Autodesk Inventor part; units mm, degrees
ref_plane "YZ Plane" through (0, 0, 0) normal (1, 0, 0) x (0, 1, 0)
ref_plane "XZ Plane" through (0, 0, 0) normal (0, 1, 0) x (-1, 0, 0)
ref_plane "XY Plane" through (0, 0, 0) normal (0, 0, 1) x (1, 0, 0)
sketch "Sketch51" plane through (0, 0, 0) normal (0, 1, 0) x (-1, 0, 0)
  line L0 (1.3484, 37.0338) -> (-3.7316, 37.0338)
  line L1 (-3.7316, 37.0338) -> (-3.7316, -191.5662)
  line L2 (-3.7316, -191.5662) -> (1.3484, -191.5662)
  line L3 (1.3484, -191.5662) -> (1.3484, 37.0338)
  point P0 (0, 0)
  dimension "d172" = 5.08
  dimension "d173" = 228.6
extrude "Extrusion37" add sketch "Sketch51" along normal blind 71.12
sketch "Sketch52" plane through (-1.3484, 0, 37.0338) normal (0, 0, 1) x (1, 0, 0)
  line L0 (5.08, 0) -> (5.08, 71.12)
  line L1 (5.08, 71.12) -> (-24.13, 71.12)
  line L2 (-24.13, 71.12) -> (-24.13, 66.04)
  line L3 (-24.13, 66.04) -> (5.08, 66.04)
  line L4 (5.08, 66.04) -> (5.08, 71.12)
  point P0 (1.3484, 0)
  dimension "d176" = 5.08
  dimension "d177" = 29.21
extrude "Extrusion38" add sketch "Sketch52" against normal blind 228.6
sketch "Sketch54" plane through (0, 0, 0) normal (0, -1, 0) x (1, 0, 0)
  line L0 (-20.3984, 37.0338) -> (-141.0484, 37.0338)
  line L1 (-141.0484, 37.0338) -> (-141.0484, -191.5662)
  line L2 (-141.0484, -191.5662) -> (-20.3984, -191.5662)
  line L3 (-20.3984, -191.5662) -> (-20.3984, 37.0338)
  line L4 (-25.4784, 37.0338) -> (-1.3484, 37.0338)
  line L5 (-1.3484, -191.5662) -> (-25.4784, -191.5662)
  line L6 (-1.3484, -191.5662) -> (-1.3484, 37.0338)
  point P0 (0, 0)
  dimension "d180" = 0
  dimension "d181" = 0
  dimension "d182" = 19.05
  dimension "d183" = 120.65
extrude "Extrusion39" add sketch "Sketch54" against normal blind 5.08 contours L3 L2 L1 L0
sketch "Sketch55" plane through (-1.3484, 0, 37.0338) normal (0, 0, 1) x (1, 0, 0)
  line L0 (-139.7, 5.08) -> (-19.05, 5.08)
  line L1 (-24.13, 66.04) -> (-24.13, 71.12)
  line L2 (-19.05, 5.08) -> (-24.13, 5.08)
  line L3 (-24.13, 5.08) -> (-24.13, 71.12)
  line L4 (-24.13, 71.12) -> (-19.05, 71.12)
  line L5 (-19.05, 71.12) -> (-19.05, 5.08)
  point P0 (1.3484, 0)
extrude "Extrusion40" add sketch "Sketch55" against normal blind 228.6
sketch "Sketch56" plane through (3.7316, 0, 37.0338) normal (0, 0, 1) x (1, 0, 0)
  line L0 (-29.4089, 71.12) -> (0, 71.12)
  line L1 (0, 71.12) -> (0, 0)
  line L2 (0, 0) -> (-29.4089, 0)
  line L3 (-29.4089, 0) -> (-29.4089, 71.12)
  line L4 (0, 71.12) -> (-29.21, 71.12)
  point P0 (-3.7316, 0)
  dimension "d275" = 0
extrude "Extrusion41" add sketch "Sketch56" against normal blind 5.08
sketch "Sketch57" plane through (3.7316, 0, -191.5662) normal (0, 0, -1) x (-1, 0, 0)
  line L0 (29.4089, 5.08) -> (29.4089, 71.12)
  line L1 (29.4089, 71.12) -> (0, 71.12)
  line L2 (0, 71.12) -> (0, -0.0331)
  line L3 (0, -0.0331) -> (29.4089, -0.0331)
  line L4 (29.4089, -0.0331) -> (29.4089, 71.12)
  point P0 (3.7316, 0)
extrude "Extrusion42" add sketch "Sketch57" against normal blind 5.08
sketch "Sketch58" plane through (0, 71.12, 0) normal (0, 1, 0) x (1, 0, 0)
  line L0 (-25.4784, -31.9538) -> (-25.4784, 186.4862)
  line L1 (-141.0484, 191.5662) -> (-141.0484, -37.0338)
  line L2 (-25.4784, 109.0162) -> (-141.0484, 109.0162)
  line L3 (-141.0484, 109.0162) -> (-141.0484, 147.1162)
  line L4 (-141.0484, 147.1162) -> (-25.4784, 147.1162)
  line L5 (-25.4784, 147.1162) -> (-25.4784, 109.0162)
  line L6 (-25.6773, 191.5662) -> (-141.0484, 191.5662)
  point P0 (0, 0)
  dimension "d192" = 38.1
  dimension "d193" = 44.45
extrude "Extrusion43" add sketch "Sketch58" against normal blind 5.08
sketch "Sketch59" plane through (-141.0484, 71.12, -147.1162) normal (-1, 0, 0) x (0, 0, 1)
  line L0 (0, 0) -> (0, -5.08)
  line L1 (184.15, -71.12) -> (-44.45, -71.12)
  line L2 (0, 0) -> (5.08, 0)
  line L3 (5.08, 0) -> (5.08, -71.12)
  line L4 (5.08, -71.12) -> (0, -71.12)
  line L5 (0, -71.12) -> (0, 0)
  line L6 (38.1, 0) -> (38.1, -5.08)
  line L7 (38.1, 0) -> (33.02, 0)
  line L8 (33.02, 0) -> (33.02, -71.12)
  line L9 (33.02, -71.12) -> (38.1, -71.12)
  line L10 (38.1, -71.12) -> (38.1, 0)
  point P0 (147.1162, -71.12)
  dimension "d196" = 5.08
  dimension "d197" = 5.08
extrude "Extrusion44" add sketch "Sketch59" against normal blind 120.65
sketch "Sketch60" plane through (-141.0484, 0, -191.5662) normal (-1, 0, 0) x (0, 0, 1)
  line L0 (49.53, 5.08) -> (77.47, 5.08)
  line L1 (5.08, 0) -> (223.52, 0)
  line L2 (49.53, 5.08) -> (77.4104, 5.08)
  line L3 (77.4104, 5.08) -> (77.4104, 0)
  line L4 (77.4104, 0) -> (49.53, 0)
  line L5 (49.53, 0) -> (49.53, 5.08)
  point P0 (191.5662, 0)
extrude "Extrusion45" cut sketch "Sketch60" against normal blind 120.65
sketch "Sketch61" plane through (-25.4784, 66.04, -142.0362) normal (-1, 0, 0) x (0, 0, 1)
  line L0 (0, -66.04) -> (0, 0)
  line L1 (27.94, 0) -> (27.94, -60.96)
  line L2 (27.94, 0) -> (0, 0)
  line L3 (-44.45, -66.04) -> (173.99, -66.04)
  line L4 (0, 0) -> (27.6512, 0)
  line L5 (27.6512, 0) -> (27.6512, -66.04)
  line L6 (27.6512, -66.04) -> (0, -66.04)
  line L7 (0, -66.04) -> (0, 0)
  point P0 (142.0362, -66.04)
extrude "Extrusion46" cut sketch "Sketch61" against normal blind 5.08
sketch "Sketch62" plane through (-141.0484, 5.08, -109.0162) normal (-1, 0, 0) x (0, 0, 1)
  line L0 (-33.02, -5.08) -> (-82.55, -5.08)
  line L1 (-38.1, 66.04) -> (-38.1, 0)
  line L2 (0, 66.04) -> (0, 0)
  line L3 (-5.1396, 0) -> (-5.1396, -5.08)
  line L4 (146.05, -5.08) -> (-5.1396, -5.08)
  line L5 (146.05, -5.08) -> (146.05, 0)
  line L6 (0, 0) -> (146.05, 0)
  line L7 (0, 66.04) -> (0, 0)
  line L8 (0, 66.04) -> (-38.1, 66.04)
  line L9 (-38.1, 66.04) -> (-38.1, 0)
  line L10 (-82.55, 0) -> (-38.1, 0)
  line L11 (-82.55, -5.08) -> (-82.55, 0)
  line L12 (-33.02, -5.08) -> (-82.55, -5.08)
  line L13 (-33.02, -5.08) -> (-33.02, 60.96)
  line L14 (-5.08, 60.96) -> (-33.02, 60.96)
  line L15 (-5.08, 60.96) -> (-5.08, 0)
  line L16 (0, 66.04) -> (-34.1859, 66.04)
  line L17 (-34.1859, 66.04) -> (-34.1859, -5.08)
  line L18 (-34.1859, -5.08) -> (0, -5.08)
  line L19 (0, -5.08) -> (0, 66.04)
  line L20 (-5.1396, 0) -> (-5.08, 0)
  point P0 (109.0162, -5.08)
extrude "Extrusion47" add sketch "Sketch62" against normal blind 5.08 contours L0 L17 L8 L2 L19 L4 L3 L20 L15 L14 L13 | L13 L14 L15 L20 L3 L18
sketch "Sketch63" plane through (3.7316, 0, -191.5662) normal (0, 0, -1) x (-1, 0, 0)
  line L0 (144.78, 0) -> (29.4089, 0)
  line L1 (29.4089, 5.08) -> (29.4089, 71.12)
  point P0 (3.7316, 0)
  point P1 (14.1689, 25.4)
  point P2 (0, 0)
  dimension "d206" = 25.4
  dimension "d207" = 15.24
hole "Hole8" at (-10.4373, 25.4, -191.5662) direction (0, 0, 1) diameter 3.302 end through all
sketch "Sketch64" plane through (-141.0484, 0, -191.5662) normal (-1, 0, 0) x (0, 0, 1)
  line L0 (228.6, 0) -> (0, 0)
  line L1 (44.45, 71.12) -> (44.45, 5.08)
  point P0 (191.5662, 0)
  point P1 (63.5, 25.4)
  dimension "d215" = 25.4
  dimension "d216" = 19.05
hole "Hole9" at (-141.0484, 25.4, -128.0662) direction (1, 0, 0) diameter 3.302 depth 25.4 tip angle 118.188
sketch "Sketch66" plane through (0, 71.12, 0) normal (0, 1, 0) x (1, 0, 0)
  line L0 (-141.0484, 109.0162) -> (-141.0484, 147.1162)
  line L1 (-25.4784, 109.0162) -> (-141.0484, 109.0162)
  line L2 (-141.0484, 147.1162) -> (-25.4784, 147.1162)
  point P0 (0, 0)
  point P1 (-77.5484, 137.5912)
  dimension "d227" = 9.525
hole "Hole10" at (-77.5484, 71.12, -137.5912) direction (0, -1, 0) diameter 3.81 depth 25.4 tip angle 118.188
sketch "Sketch69" plane through (-141.0484, 71.12, -109.0162) normal (0, 0, 1) x (1, 0, 0)
  line L0 (31.75, -38.1) -> (83.6211, -38.1) construction
  line L1 (31.75, -19.05) -> (83.6211, -19.05)
  line L2 (83.6211, -57.15) -> (31.75, -57.15)
  arc A0 (31.75, -19.05) -> (31.75, -57.15) centre (31.75, -38.1) ccw
  arc A1 (83.6211, -57.15) -> (83.6211, -19.05) centre (83.6211, -38.1) ccw
  line L3 (0, 0) -> (0, -66.04)
  line L4 (115.3711, -66.04) -> (115.3711, 0)
  line L5 (115.57, 0) -> (0, 0)
  point P0 (141.0484, -71.12)
  point P1 (57.6856, -38.1)
  dimension "d252" = 31.75
  dimension "d253" = 31.75
  dimension "d254" = 38.1
  dimension "d255" = 19.05
extrude "Extrusion49" cut sketch "Sketch69" against normal blind 230.1875
sketch "Sketch70" plane through (0, 71.12, 0) normal (0, 1, 0) x (1, 0, 0)
  line L0 (-20.3984, -31.9538) -> (-20.3984, 114.385)
  line L1 (-25.4784, -31.9538) -> (-25.4784, 109.0162)
  line L2 (-25.4784, 109.0162) -> (-141.0484, 109.0162)
  line L3 (-141.0484, 191.5662) -> (-141.0484, -37.0338)
  line L4 (-141.0484, -37.0338) -> (-25.6773, -37.0338)
  line L5 (-141.0484, 109.0162) -> (-141.0484, 147.1162)
  line L6 (-141.0484, 109.0162) -> (-25.6773, 109.0162)
  line L7 (-25.6773, 109.0162) -> (-25.6773, -37.0338)
  line L8 (-25.6773, -37.0338) -> (-141.0484, -37.0338)
  line L9 (-141.0484, -37.0338) -> (-141.0484, 109.0162)
  point P0 (0, 0)
extrude "Extrusion50" add sketch "Sketch70" against normal blind 15.24
sketch "Sketch71" plane through (0, 71.12, 0) normal (0, 1, 0) x (1, 0, 0)
  line L0 (-25.6773, -37.0338) -> (3.7316, -37.0338)
  line L1 (3.7316, -37.0338) -> (-155.1721, -37.0338)
  line L2 (-155.1721, -37.0338) -> (-155.1721, 120.4462)
  line L3 (-155.1721, 120.4462) -> (3.7316, 120.4462)
  line L4 (3.7316, 120.4462) -> (3.7316, -37.0338)
  point P0 (0, 0)
  dimension "d260" = 157.48
extrude "Extrusion51" cut sketch "Sketch71" against normal blind 5.08
sketch "Sketch72" plane through (0, 66.04, 0) normal (0, 1, 0) x (1, 0, 0)
  line L0 (3.7316, -37.0338) -> (3.7316, -31.9538)
  line L1 (3.7316, -37.0338) -> (-25.8998, -37.0338)
  line L2 (-25.8998, -37.0338) -> (-25.8998, 126.8083)
  line L3 (-25.8998, 126.8083) -> (3.7316, 126.8083)
  line L4 (3.7316, 126.8083) -> (3.7316, -37.0338)
  point P0 (0, 0)
extrude "Extrusion52" add sketch "Sketch72" against normal blind 5.08
sketch "Sketch73" plane through (0, 66.04, 0) normal (0, 1, 0) x (1, 0, 0)
  line L0 (-137.7579, 102.3229) -> (-23.4148, 102.3229)
  line L1 (-23.4148, 102.3229) -> (-23.4148, 125.8312)
  line L2 (-23.4148, 125.8312) -> (-137.7579, 125.8312)
  line L3 (-137.7579, 125.8312) -> (-137.7579, 102.3229)
  point P0 (0, 0)
extrude "Extrusion53" add sketch "Sketch73" against normal blind 5.08
sketch "Sketch74" plane through (0, 66.04, 0) normal (0, 1, 0) x (1, 0, 0)
  line L0 (-141.0484, -37.0338) -> (-141.0484, 120.4462)
  line L1 (-141.0484, -37.0338) -> (-52.1484, -37.0338)
  line L2 (-52.1484, -37.0338) -> (-52.1484, 64.5662)
  line L3 (-52.1484, 64.5662) -> (-141.0484, 64.5662)
  line L4 (-141.0484, 64.5662) -> (-141.0484, -37.0338)
  point P0 (0, 0)
  dimension "d267" = 88.9
  dimension "d268" = 101.6
extrude "Extrusion54" cut sketch "Sketch74" against normal blind 37.7825
sketch "Sketch76" plane through (-141.0484, 0, -191.5662) normal (-1, 0, 0) x (0, 0, 1)
  line L0 (82.55, 55.88) -> (82.55, 5.08)
  line L1 (127, 55.88) -> (82.55, 55.88)
  line L2 (82.55, 55.88) -> (127, 55.88)
  line L3 (127, 55.88) -> (82.55, 51.6083)
  line L4 (82.55, 51.6083) -> (82.55, 55.88)
  point P0 (191.5662, 0)
extrude "Extrusion55" add sketch "Sketch76" against normal blind 116.205
sketch "Sketch77" plane through (-141.0484, 0, 37.0338) normal (0, 0, 1) x (1, 0, 0)
  line L0 (115.3711, 55.88) -> (88.9, 55.88)
  line L1 (115.3711, 5.08) -> (115.3711, 55.88)
  line L2 (88.9, 55.88) -> (0, 55.88)
  line L3 (88.9, 55.88) -> (115.3711, 55.88)
  line L4 (115.3711, 47.4297) -> (88.9, 55.88)
  point P0 (141.0484, 0)
extrude "Extrusion56" add sketch "Sketch77" against normal blind 158.4325
sketch "Sketch78" plane through (0, 5.08, 0) normal (0, 1, 0) x (1, 0, 0)
  line L0 (-141.0484, -37.0338) -> (-25.6773, -37.0338)
  line L1 (-141.0484, 109.0162) -> (-141.0484, -37.0338)
  point P0 (0, 0)
  point P1 (-90.2484, 26.4662)
  dimension "d276" = 63.5
  dimension "d277" = 50.8
hole "Hole12" at (-90.2484, 5.08, -26.4662) direction (0, -1, 0) diameter 3.81 depth 25.4 tip angle 118.188
equation "\"d172\" = WallWidth"
equation "\"d173\" = PartLength"
equation "\"d174\" = CPDeckHeight"
equation "\"d176\" = WallWidth"
equation "\"d177\" = 2 * WallWidth + ControlPlateShelfLength"
equation "\"d178\" = PartLength"
equation "\"d182\" = ControlPlateShelfLength"
equation "\"d183\" = CPDWidthHole"
equation "\"d184\" = WallWidth"
equation "\"d186\" = PartLength"
equation "\"d188\" = WallWidth"
equation "\"d190\" = WallWidth"
equation "\"d194\" = WallWidth"
equation "\"d196\" = WallWidth"
equation "\"d197\" = WallWidth"
equation "\"d202\" = WallWidth"
equation "\"d204\" = WallWidth"
equation "\"d261\" = WallWidth"
equation "\"d263\" = WallWidth"
equation "\"d265\" = WallWidth"
equation "\"DSLength\" = 1371.6"
equation "\"DSWidth\" = 304.8"
equation "\"DCDeckHeight\" = 76.2"
equation "\"WallWidth\" = 5.08"
equation "\"EdgeAngle\" = 10deg"
equation "\"LengthCuts\" = 152.4"
equation "\"WidthCuts\" = 50.8"
equation "\"PartLength\" = 228.6"
equation "\"PartWidth\" = 152.4"
equation "\"BoltHoldDiam\" = 6.35"
equation "\"ControlPlateLength\" = 228.6"
equation "\"ControlPlateWidth\" = 228.6"
equation "\"ControlPlateShelfLength\" = 19.05"
equation "\"ControlHoleLength\" = 190.5"
equation "\"ControlHoleWidth\" = 190.5"
equation "\"ControlHoleFromSide\" = 63.5"
equation "\"ControlHoleBoltHoleMid\" = 9.525"
equation "\"CPDeckHeight\" = 71.12"
equation "\"CPFromSide\" = 63.5"
equation "\"CPFromBack\" = 63.5"
equation "\"DU1CHWidth\" = 69.85"
equation "\"DU1CHLength\" = 146.05"
equation "\"ControlPlateScrewLength\" = 76.2"
equation "\"DSBackHeight\" = 127"
equation "\"BackShelf\" = 25.4"
equation "\"MainAngle\" = 168.22deg"
equation "\"CPDWidthHole\" = 120.65"
equation "\"CPDLengthHole\" = 146.05"
equation "\"DownBackHeight\" = 130.7084"
properties part number "CPLRightThree"
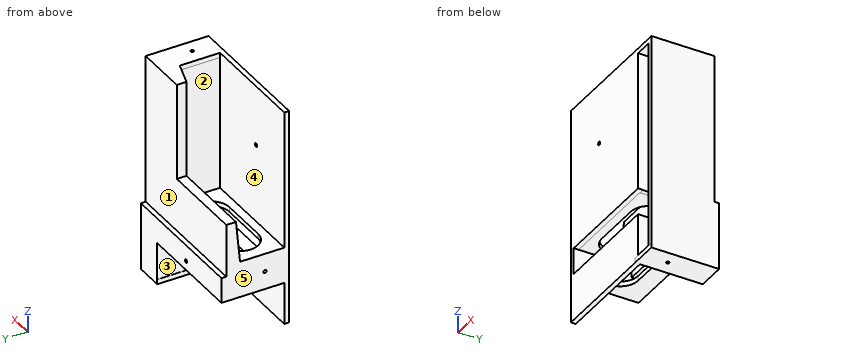
Geometry: final body of the model. Coordinates: model frame, mm. Face numbers are marked on the shaded views. A direction names the side the tool comes from. Coordinates: 2 decimals unless noted, no trailing zeros. Order: outer loops, then holes, each group sorted by start corner. A loop starts at its lowest first (then second) coordinate and runs counter-clockwise, first axis right, second up. Notation, with made-up numbers: (60.25, 86) -> (84.25, 86) arc R21 ccw to (84.25, 103) -> close; hole circle Ø2 at (57.25, -27.75). An arc over 180 degrees is marked (long way). Answer in a Markdown table with one row per item.
Item 1: Access query for the marked faces 4 and 5. Directions: +Z, -Z, +X, -X, +Y, -Y. A direction counts if a zero-diameter tool reaches every point of the face in a straight line with its end or side. Return the directions, or none.
Return value:
| item | result |
|---|---|
| face 4 | +Z, -X |
| face 5 | +Z, -Z, -X, +Y, -Y |
Item 2: Draft query along Y for the marked faces 1, 2 and 3. Return one class per face: released by +Y, released by -Y, zero draft, split by the parting line, or undercut.
Return value:
| item | result |
|---|---|
| face 1 | released by +Y |
| face 2 | undercut |
| face 3 | zero draft |
Item 3: Section C-C on z = -170. Output: boundary loops of the cut face in (x, y), plus the area to 3 significant figures.
Return value:
| item | result |
|---|---|
| outline | (-141.05, 0) -> (-20.4, 0) -> (-20.4, 66.04) -> (-1.35, 66.04) -> (-1.35, 0) -> (3.73, 0) -> (3.73, 71.12) -> (-25.48, 71.12) -> (-25.48, 5.08) -> (-141.05, 5.08) -> close |
| area | 1,410 mm² |
Item 4: Contact query for flat-ended pins moving along their axis: P1, Ø1.5, axis at y = 13.5, z = -23.5, coming from the -X side; P2, Ø1.5, axis at x = -91, z = -81, coming from the -Y side; P3, Ø2.5, axis at x = -52, y = 68.5, coming from the +Z side; P4, Ø4.5, axis at x = -77.55, z = -137.59, coming from the +Y side. Output: stop coordinate, or through.
Return value:
| item | result |
|---|---|
| P1 | stops at x = -25.48 |
| P2 | stops at y = 0 |
| P3 | stops at z = -120.45 |
| P4 | stops at y = 71.12 |
Item 5: Section D-D on z = -88.5. Output: boundary loops of the cut face in (x, y).
Return value:
| item | result |
|---|---|
| outline | (-141.05, 0) -> (-20.4, 0) -> (-20.4, 60.96) -> (-1.35, 60.96) -> (-1.35, 0) -> (3.73, 0) -> (3.73, 66.04) -> (-141.05, 66.04) -> (-141.05, 53.58) -> (-44.94, 53.58) -> (-25.68, 47.43) -> (-25.68, 53.58) -> (-25.48, 53.58) -> (-25.48, 5.08) -> (-141.05, 5.08) -> close; hole (-25.68, 55.88) -> (-25.48, 55.88) -> (-25.48, 60.96) -> (-25.68, 60.96) -> close |
Item 6: Section B-B on x = -86. Output: boundary loops of the cut face in (y, z), plus the area to 3 significant figures.
Return value:
| item | result |
|---|---|
| outline | (0, -191.57) -> (5.08, -191.57) -> (5.08, -147.12) -> (13.97, -147.12) -> (13.97, -142.04) -> (0, -142.04) -> close; (0, -114.16) -> (5.08, -114.16) -> (5.08, -114.1) -> (13.97, -114.1) -> (13.97, -109.02) -> (5.08, -109.02) -> (5.08, 37.03) -> (0, 37.03) -> close; (51.61, -109.02) -> (52.07, -109.02) -> (52.07, -114.1) -> (60.96, -114.1) -> (60.96, -125.83) -> (66.04, -125.83) -> (66.04, -142.04) -> (52.07, -142.04) -> (52.07, -147.12) -> (71.12, -147.12) -> (71.12, -120.45) -> (66.04, -120.45) -> (66.04, -64.57) -> (55.88, -64.57) -> close |
| area | 1,990 mm² |
Item 7: Ray query, L1, parallel to Z at x = -140, y = 25.4; L2, parallel to Z at x = -129.5, y = 44; L3, parallel to X at y = 25.4, z = -188.1. Return the intervals inside material, ascending.
Return value:
| item | result |
|---|---|
| L1 | z = -147.12 to -129.72, -126.42 to -109.02 |
| L2 | z = -147.12 to -142.04, -114.1 to -109.02 |
| L3 | x = -25.68 to -12.09, -8.79 to 3.73 |
